```python
from build123d import *

# Parameters (mm, degrees)
SKETCH1_W           = 85
SKETCH1_H           = 70
BOSS_EXTRUDE1_DEPTH = 3
SKETCH2_R           = 1.25
CUT_EXTRUDE1_DEPTH  = 56.138462075
SKETCH3_W           = 20
SKETCH3_H           = 3
BOSS_EXTRUDE2_DEPTH = 3
SKETCH4_R           = 1.5
CUT_EXTRUDE2_DEPTH  = 10
CUT_EXTRUDE3_DEPTH  = 10
FILLET1_R           = 1
SKETCH6_W           = 16.5
SKETCH6_H           = 14
CUT_EXTRUDE4_DEPTH  = 58.089841478
FILLET2_R           = 1
SKETCH11_R          = 3
CUT_EXTRUDE9_DEPTH  = 10


with BuildPart() as part:
    # Sketch1 → Boss-Extrude1 (new body)
    with BuildSketch(Plane(origin=(0, 0, 0), x_dir=(1, 0, 0), z_dir=(0, 1, 0))):
        Rectangle(SKETCH1_W, SKETCH1_H)
    extrude(amount=BOSS_EXTRUDE1_DEPTH)

    # Sketch2 → Cut-Extrude1 (cut, through all)
    with BuildSketch(Plane(origin=(0, 3, 0), x_dir=(1, 0, 0), z_dir=(0, 1, 0))):
        with Locations(Location((-38.5, 24, 0), (0, 0, 270))):
            Circle(SKETCH2_R)
        with Locations(Location((-38.5, -25, 0), (0, 0, 270))):
            Circle(SKETCH2_R)
        with Locations(Location((19.5, -25, 0), (0, 0, 270))):
            Circle(SKETCH2_R)
        with Locations(Location((19.5, 24, 0), (0, 0, 270))):
            Circle(SKETCH2_R)
    extrude(amount=-CUT_EXTRUDE1_DEPTH, mode=Mode.SUBTRACT)

    # Sketch3 → Boss-Extrude2 (add)
    with BuildSketch(Plane(origin=(0, 3, 0), x_dir=(1, 0, 0), z_dir=(0, 1, 0))):
        with Locations((-22.5, 36.5)):
            Rectangle(SKETCH3_W, SKETCH3_H)
        with Locations((22.5, 36.5)):
            Rectangle(SKETCH3_W, SKETCH3_H)
        with Locations((22.5, -36.5)):
            Rectangle(SKETCH3_W, SKETCH3_H)
        with Locations((-22.5, -36.5)):
            Rectangle(SKETCH3_W, SKETCH3_H)
    extrude(amount=-BOSS_EXTRUDE2_DEPTH)

    # Sketch4 → Cut-Extrude2 (cut)
    with BuildSketch(Plane(origin=(0, 3, 0), x_dir=(1, 0, 0), z_dir=(0, 1, 0))):
        with Locations(Location((-39.5, -32, 0), (0, 0, 270))):
            Circle(SKETCH4_R)
        with Locations(Location((39.5, -32, 0), (0, 0, 270))):
            Circle(SKETCH4_R)
        with Locations(Location((39.5, 32, 0), (0, 0, 270))):
            Circle(SKETCH4_R)
        with Locations(Location((-39.5, 32, 0), (0, 0, 270))):
            Circle(SKETCH4_R)
    extrude(amount=-CUT_EXTRUDE2_DEPTH, mode=Mode.SUBTRACT)

    # Sketch5 → Cut-Extrude3 (cut)
    with BuildSketch(Plane(origin=(0, 3, 0), x_dir=(1, 0, 0), z_dir=(0, 1, 0))):
        Polygon((-34, 27.5), (-34, 19.5), (-39, 19.5), (-39, -20.5), (-34, -20.5), (-34, -28.5), (15, -28.5), (15, -20.5), (23, -20.5), (23, 19.5), (15, 19.5), (15, 27.5), align=None)
    extrude(amount=-CUT_EXTRUDE3_DEPTH, mode=Mode.SUBTRACT)

    # Fillet1
    fillet1_edges = [part.edges().sort_by_distance(p)[0] for p in [
        (-34, 1.5, 20.5),
        (-39, 1.5, 20.5),
        (-39, 1.5, -19.5),
        (-34, 1.5, -19.5),
        (-34, 1.5, -27.5),
        (15, 1.5, -27.5),
        (15, 1.5, -19.5),
        (23, 1.5, -19.5),
        (23, 1.5, 20.5),
        (15, 1.5, 20.5),
        (15, 1.5, 28.5),
        (-34, 1.5, 28.5),
    ]]
    fillet(fillet1_edges, radius=FILLET1_R)

    # Sketch6 → Cut-Extrude4 (cut, through all)
    with BuildSketch(Plane(origin=(0, 3, 0), x_dir=(1, 0, 0), z_dir=(0, 1, 0))):
        with Locations((31.25, -0.5)):
            Rectangle(SKETCH6_W, SKETCH6_H)
    extrude(amount=-CUT_EXTRUDE4_DEPTH, mode=Mode.SUBTRACT)

    # Fillet2
    fillet2_edges = [part.edges().sort_by_distance(p)[0] for p in [
        (23, 1.5, 7.5),
        (23, 1.5, -6.5),
        (39.5, 1.5, -6.5),
        (39.5, 1.5, 7.5),
    ]]
    fillet(fillet2_edges, radius=FILLET2_R)

    # Sketch11 → Cut-Extrude9 (cut)
    with BuildSketch(Plane(origin=(0, 3, 0), x_dir=(1, 0, 0), z_dir=(0, 1, 0))):
        with Locations(Location((27, -20, 0), (0, 0, 270))):
            Circle(SKETCH11_R)
    extrude(amount=-CUT_EXTRUDE9_DEPTH, mode=Mode.SUBTRACT)


solid = part.part
```
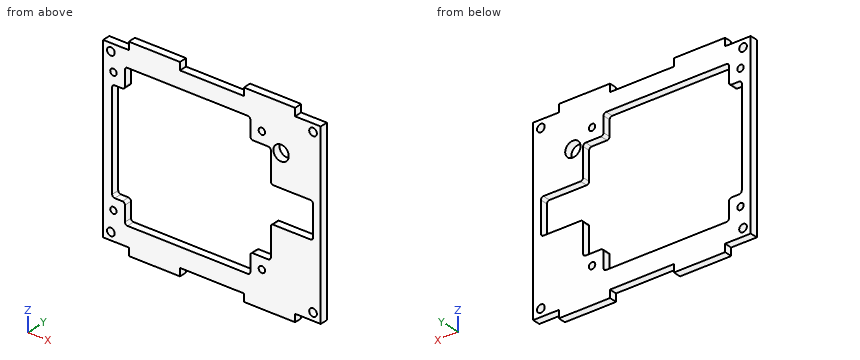
The listing builds one solid part. Answer for the finished solid, in the listing's coordinates (mm). Give positions to 0.01 mm unless a question says otherwise; leave off trailing zeros. Order: outer loops, then holes, each group sorted by start corner. A loop starts at its lowest first (then second) coordinate and runs counter-clockwise, first axis right, second up. Notation, with made-up numbers: (70.5, -19) - (98.5, -19) arc R24 ccw to (98.5, 1) - close; hole circle Ø2 at (-5, 36). An arc over 180 degrees is marked (long way). Answer in a Markdown table with one row per item. Add a question column.
Q1. Find the intervals of material crossed by line 1 along X through (y, z) = (1.85, 32); line 2 along X through (y, z) = (1.05, -24); line 3 along Z through (x, y) = (30.5, 1.45), in increasing order. Write a range as [from, to].
Q2. The part is cut by section B-B (x = -5). Determine the outline of the cut face in (y, z).
Q3. The part is cut by section A-A (z = 32). Determine the outline of the cut face in (x, y).
Q4. The part is cut by section D-D (z = -24). Determine the outline of the cut face in (x, y).
Q5. The part is cut by section C-C (x = 19.5). Determine the outline of the cut face in (y, z).
Q6. Given P1, Ø1.5, axis at x = 11.5, y = 2.5, coming from the -Z side; P2, Ø1.5, axis at x = -39.5, y = 1.5, coming from the +Z side; P3, Ø1.5, axis at y = 1.5, z = 36.5, coming from the +X side, each flat-ended and moving along its own axis, determine where each tip first touches the part or whether it passes through.
Determined:
| question | item | result |
|---|---|---|
| 1 | line 1 | x = [-42.5, -41], [-38, 38], [41, 42.5] |
| 1 | line 2 | x = [-42.5, -39.75], [-37.25, -34], [15, 18.25], [20.75, 42.5] |
| 1 | line 3 | z = [-38, -6.5], [7.5, 38] |
| 2 | outline | (0, -35) - (3, -35) - (3, -27.5) - (0, -27.5) - close; (0, 28.5) - (3, 28.5) - (3, 35) - (0, 35) - close |
| 3 | outline | (-42.5, 0) - (-41, 0) - (-41, 3) - (-42.5, 3) - close; (-38, 0) - (38, 0) - (38, 3) - (-38, 3) - close; (41, 0) - (42.5, 0) - (42.5, 3) - (41, 3) - close |
| 4 | outline | (-42.5, 0) - (-39.75, 0) - (-39.75, 3) - (-42.5, 3) - close; (-37.25, 0) - (-34, 0) - (-34, 3) - (-37.25, 3) - close; (15, 0) - (18.25, 0) - (18.25, 3) - (15, 3) - close; (20.75, 0) - (42.5, 0) - (42.5, 3) - (20.75, 3) - close |
| 5 | outline | (0, -38) - (3, -38) - (3, -25.25) - (0, -25.25) - close; (0, -22.75) - (3, -22.75) - (3, -19.5) - (0, -19.5) - close; (0, 20.5) - (3, 20.5) - (3, 23.75) - (0, 23.75) - close; (0, 26.25) - (3, 26.25) - (3, 38) - (0, 38) - close |
| 6 | P1 | stops at z = -35 |
| 6 | P2 | stops at z = 35 |
| 6 | P3 | stops at x = 32.5 |
